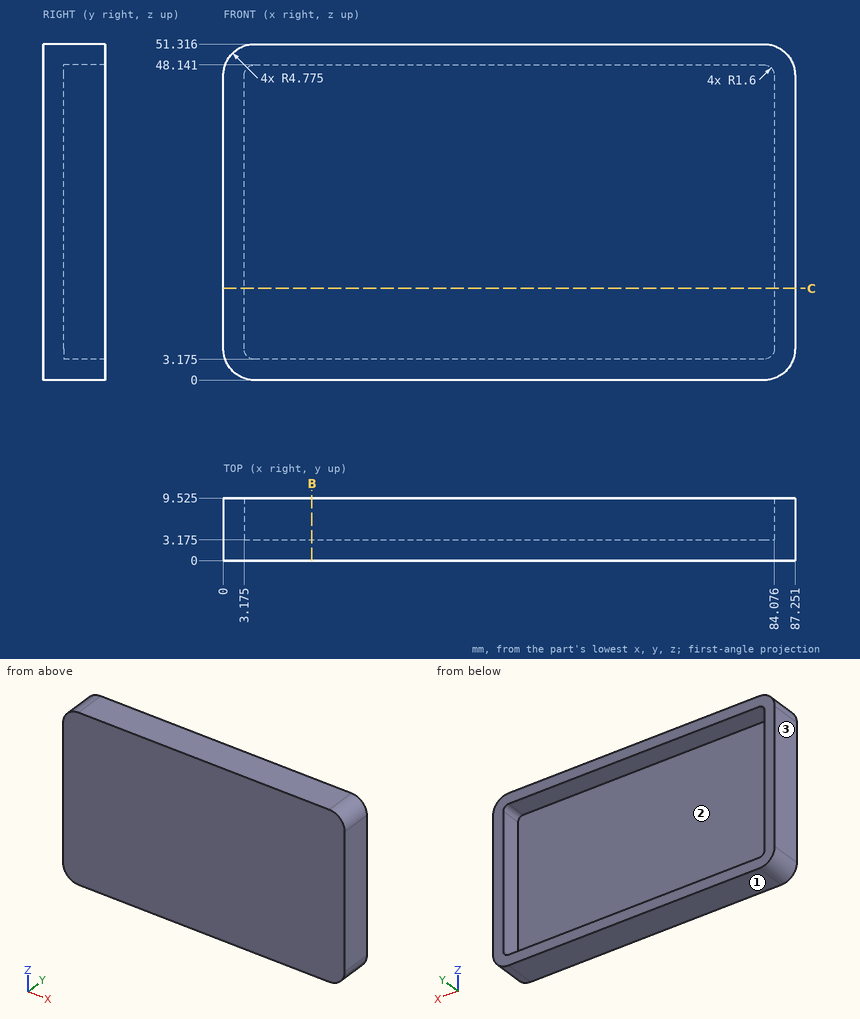
Verification items for this drawing (mm, ordinates from the low corner). Round coordinates to 2 decimals unless told otherwise and drop trailing zeros. Loops run counter-clockwise (first coordinate to the right, second up) from the corner with the lowest first, then second, coordinate; pieces in that order, holes last. Notation, with made-up numbers: (75, -9) - (113, -9) arc R28 cw to (113, 23) - close; hole circle Ø8 at (-28.5, 38). An arc over 180 degrees is marked (long way). Answer as CSV lines item,"result". Start each with the question number.
Item 1: Scan lines: line 1 (X direction, y = 4.5, z = 42.5) (1 decimal); line 2 (Z direction, x = 78.5, y = 7.5) (1 decimal); line 3 (Y direction, x = 4.5, z = 40.5) (3 decimals). Record each from-to range of solid material in increasing order. Write a range as [from, to].
Item 2: Depth check by flat-ended pin: P1, Ø1.9, axis at x = 35, y = 5.5, coming from the -Z side; P2, Ø3, axis at x = 57, z = 7.5, coming from the +Y side (3 decimals). Enter the tip coordinate at first touch or a pass-through.
Item 3: Section check C-C (z = 14). Record the boundary of the cut face in (x, y) (1 decimal).
Item 4: Release check for a two-part mould opening along Z. For the marked faces 1, 2 and 3 record: +Z half, -Z half, draft (parallel to the pull), parting line (faces both ways), or undercut.
Item 5: Section check B-B (x = 13.5). Record the boundary of the cut face in (y, z) (1 decimal).
Report:
1,line 1,"x = [0, 3.2], [84.1, 87.3]"
1,line 2,"z = [0, 3.2], [48.1, 51.3]"
1,line 3,"y = [0, 3.175]"
2,P1,"stops at z = 0"
2,P2,"stops at y = 3.175"
3,outline,"(0, 0) - (87.3, 0) - (87.3, 9.5) - (84.1, 9.5) - (84.1, 3.2) - (3.2, 3.2) - (3.2, 9.5) - (0, 9.5) - close"
4,face 1,"-Z half"
4,face 2,"undercut"
4,face 3,"draft"
5,outline,"(0, 0) - (9.5, 0) - (9.5, 3.2) - (3.2, 3.2) - (3.2, 48.1) - (9.5, 48.1) - (9.5, 51.3) - (0, 51.3) - close"
